Build history of the part. All positions in model axes, mm. A direction names the side the tool comes from. Give positions to 0.01 mm unless a question says otherwise; leave off trailing zeros. Write each loop counter-clockwise with the first axis right and the second up, starting at its lowest first coordinate (ties: lowest second). Pieces come first, ordered by that corner, then holes.
from build123d import *

# Parameters (mm, degrees)
SKETCH1_R                       = 1.5
BOSS_EXTRUDE1_DEPTH             = 2
SKETCH2_W                       = 4
SKETCH2_H                       = 25
BOSS_EXTRUDE2_DEPTH             = 15
FILLET1_R                       = 12.5
SKETCH3_R                       = 1.75
CUT_EXTRUDE3_DEPTH              = 53.391713426
CIRPATTERN1_COUNT               = 4
CIRPATTERN1_ANGLE               = 90
CIRPATTERN1_THE_OTHER_WAY_COUNT = 4
CIRPATTERN1_THE_OTHER_WAY_ANGLE = 90
MIRROR1_COPY_1_SKETCH_R         = 1.75
MIRROR1_COPY_1_DEPTH            = 53.391713426
MIRROR1_COPY_2_SKETCH_R         = 1.75
MIRROR1_COPY_2_DEPTH            = 53.391713426
MIRROR1_COPY_3_SKETCH_R         = 1.75
MIRROR1_COPY_3_DEPTH            = 53.391713426
MIRROR1_COPY_4_SKETCH_R         = 1.75
MIRROR1_COPY_4_DEPTH            = 53.391713426
MIRROR1_COPY_5_SKETCH_R         = 1.75
MIRROR1_COPY_5_DEPTH            = 53.391713426
MIRROR1_COPY_6_SKETCH_R         = 1.75
MIRROR1_COPY_6_DEPTH            = 53.391713426
FILLET1_OF_MIRROR1_R            = 12.5
SKETCH4_W                       = 30.151429758
SKETCH4_H                       = 10
BOSS_EXTRUDE3_DEPTH             = 7
FILLET2_R                       = 5


with BuildPart() as part:
    # Sketch1 → Boss-Extrude1 (new body)
    with BuildSketch(Plane(origin=(0, 0, 0), x_dir=(1, 0, 0), z_dir=(0, 1, 0))):
        with BuildLine():
            Line((-17.075714879, 5.179541619), (-17.075714879, 25.179541619))
            Line((-17.075714879, 25.179541619), (-26.075714879, 25.179541619))
            ThreePointArc((-26.075714879, 25.179541619), (-26.782821661, 24.8866484), (-27.075714879, 24.179541619))
            Line((-27.075714879, 24.179541619), (-27.075714879, -25.303833099))
            ThreePointArc((-27.075714879, -25.303833099), (-26.782821661, -26.010939881), (-26.075714879, -26.303833099))
            Line((-26.075714879, -26.303833099), (25.924285121, -26.303833099))
            ThreePointArc((25.924285121, -26.303833099), (26.631391902, -26.010939881), (26.924285121, -25.303833099))
            Line((26.924285121, -25.303833099), (26.924285121, 24.179541619))
            ThreePointArc((26.924285121, 24.179541619), (26.631391902, 24.8866484), (25.924285121, 25.179541619))
            Line((25.924285121, 25.179541619), (16.924285121, 25.179541619))
            Line((16.924285121, 25.179541619), (16.924285121, 5.179541619))
            ThreePointArc((16.924285121, 5.179541619), (15.459819027, 1.644007713), (11.924285121, 0.179541619))
            Line((11.924285121, 0.179541619), (-12.075714879, 0.179541619))
            ThreePointArc((-12.075714879, 0.179541619), (-15.611248785, 1.644007713), (-17.075714879, 5.179541619))
        make_face()
        with Locations(Location((-24.075714879, 22.179541619, 0), (0, 0, 270))):
            Circle(SKETCH1_R, mode=Mode.SUBTRACT)
        with Locations(Location((23.924285121, 22.179541619, 0), (0, 0, 270))):
            Circle(SKETCH1_R, mode=Mode.SUBTRACT)
        with Locations(Location((-24.075714879, -11.220458381, 0), (0, 0, 270))):
            Circle(SKETCH1_R, mode=Mode.SUBTRACT)
        with Locations(Location((-10.075714879, -22.220458381, 0), (0, 0, 270))):
            Circle(SKETCH1_R, mode=Mode.SUBTRACT)
        with Locations(Location((9.924285121, -22.220458381, 0), (0, 0, 270))):
            Circle(SKETCH1_R, mode=Mode.SUBTRACT)
        with Locations(Location((0, -20.835125629, 0), (0, 0, 270))):
            Circle(SKETCH1_R, mode=Mode.SUBTRACT)
        with Locations(Location((23.924285121, -11.220458381, 0), (0, 0, 270))):
            Circle(SKETCH1_R, mode=Mode.SUBTRACT)
    extrude(amount=BOSS_EXTRUDE1_DEPTH)

    # Sketch2 → Boss-Extrude2 (add)
    with BuildSketch(Plane(origin=(0, 2, 0), x_dir=(1, 0, 0), z_dir=(0, 1, 0))):
        with Locations((-17.075714879, -13.803833099)):
            Rectangle(SKETCH2_W, SKETCH2_H)
    boss_extrude2 = extrude(amount=BOSS_EXTRUDE2_DEPTH)

    # Fillet1
    fillet1_edges = [part.edges().sort_by_distance(p)[0] for p in [
        (-17.075714879, 17, 26.303833099),
        (-17.075714879, 17, 1.303833099),
    ]]
    fillet(fillet1_edges, radius=FILLET1_R - 0.0001)  # a hair under: the kernel refuses the full size

    # Sketch3 → Cut-Extrude3 (cut, through all)
    with BuildSketch(Plane(origin=(-15.075714879, 0, 0), x_dir=(0, 0, -1), z_dir=(1, 0, 0))):
        with Locations((-13.803833099, 14)):
            Circle(SKETCH3_R)
    cut_extrude3 = extrude(amount=-CUT_EXTRUDE3_DEPTH, mode=Mode.SUBTRACT)

    # CirPattern1: Cut-Extrude3 ×4 about axis
    cirpattern1_axis = Axis((0, 4.5, 13.803833099), (1, 0, 0))
    for i in range(1, CIRPATTERN1_COUNT):
        add(cut_extrude3.rotate(cirpattern1_axis, i * CIRPATTERN1_ANGLE / (CIRPATTERN1_COUNT - 1)), mode=Mode.SUBTRACT)

    # CirPattern1 the other way: Cut-Extrude3 ×4 about axis
    cirpattern1_the_other_way_axis = Axis((0, 4.5, 13.803833099), (-1, 0, 0))
    for i in range(1, CIRPATTERN1_THE_OTHER_WAY_COUNT):
        add(cut_extrude3.rotate(cirpattern1_the_other_way_axis, i * CIRPATTERN1_THE_OTHER_WAY_ANGLE / (CIRPATTERN1_THE_OTHER_WAY_COUNT - 1)), mode=Mode.SUBTRACT)

    # Mirror1: Boss-Extrude2, Cut-Extrude3 across plane
    add(boss_extrude2.mirror(Plane(origin=(0, 0, 0), x_dir=(0, 0, 1), z_dir=(1, 0, 0))))
    add(cut_extrude3.mirror(Plane(origin=(0, 0, 0), x_dir=(0, 0, 1), z_dir=(1, 0, 0))), mode=Mode.SUBTRACT)

    # Mirror1 copy 1 sketch → Mirror1 copy 1 (cut, through all)
    with BuildSketch(Plane(origin=(15.075714879, 7.504802233, -0.400637034), x_dir=(0, 0.5000000000000008, -0.8660254037844382), z_dir=(-1, 0, 0))):
        with Locations((-13.803833099, -14)):
            Circle(MIRROR1_COPY_1_SKETCH_R)
    extrude(amount=-MIRROR1_COPY_1_DEPTH, mode=Mode.SUBTRACT)

    # Mirror1 copy 2 sketch → Mirror1 copy 2 (cut, through all)
    with BuildSketch(Plane(origin=(15.075714879, 14.204470134, 3.004802233), x_dir=(0, 0.8660254037844396, -0.4999999999999984), z_dir=(-1, 0, 0))):
        with Locations((-13.803833099, -14)):
            Circle(MIRROR1_COPY_2_SKETCH_R)
    extrude(amount=-MIRROR1_COPY_2_DEPTH, mode=Mode.SUBTRACT)

    # Mirror1 copy 3 sketch → Mirror1 copy 3 (cut, through all)
    with BuildSketch(Plane(origin=(15.075714879, 18.303833099, 9.303833099), x_dir=(0, 1, 0), z_dir=(-1, 0, 0))):
        with Locations((-13.803833099, -14)):
            Circle(MIRROR1_COPY_3_SKETCH_R)
    extrude(amount=-MIRROR1_COPY_3_DEPTH, mode=Mode.SUBTRACT)

    # Mirror1 copy 4 sketch → Mirror1 copy 4 (cut, through all)
    with BuildSketch(Plane(origin=(15.075714879, -6.299030867, 4.099362966), x_dir=(0, -0.5000000000000008, -0.8660254037844382), z_dir=(-1, 0, 0))):
        with Locations((-13.803833099, -14)):
            Circle(MIRROR1_COPY_4_SKETCH_R)
    extrude(amount=-MIRROR1_COPY_4_DEPTH, mode=Mode.SUBTRACT)

    # Mirror1 copy 5 sketch → Mirror1 copy 5 (cut, through all)
    with BuildSketch(Plane(origin=(15.075714879, -9.704470134, 10.799030867), x_dir=(0, -0.8660254037844396, -0.4999999999999984), z_dir=(-1, 0, 0))):
        with Locations((-13.803833099, -14)):
            Circle(MIRROR1_COPY_5_SKETCH_R)
    extrude(amount=-MIRROR1_COPY_5_DEPTH, mode=Mode.SUBTRACT)

    # Mirror1 copy 6 sketch → Mirror1 copy 6 (cut, through all)
    with BuildSketch(Plane(origin=(15.075714879, -9.303833099, 18.303833099), x_dir=(0, -1, 0), z_dir=(-1, 0, 0))):
        with Locations((-13.803833099, -14)):
            Circle(MIRROR1_COPY_6_SKETCH_R)
    extrude(amount=-MIRROR1_COPY_6_DEPTH, mode=Mode.SUBTRACT)

    # Fillet1 of Mirror1
    fillet1_of_mirror1_edges = [part.edges().sort_by_distance(p)[0] for p in [
        (17.075714879, 17, 26.303833099),
        (17.075714879, 17, 1.303833099),
    ]]
    fillet(fillet1_of_mirror1_edges, radius=FILLET1_OF_MIRROR1_R - 0.0001)  # a hair under: the kernel refuses the full size

    # Sketch4 → Boss-Extrude3 (add)
    with BuildSketch(Plane(origin=(0, 2, 0), x_dir=(1, 0, 0), z_dir=(0, 1, 0))):
        with Locations((0, -12.553833099)):
            Rectangle(SKETCH4_W, SKETCH4_H)
    extrude(amount=BOSS_EXTRUDE3_DEPTH)

    # Fillet2
    fillet2_edges = [part.edges().sort_by_distance(p)[0] for p in [
        (0, 9, 17.553833099),
        (0, 9, 7.553833099),
    ]]
    fillet(fillet2_edges, radius=FILLET2_R - 0.0001)  # a hair under: the kernel refuses the full size


solid = part.part
1. Drop flat-ended pins along their axis: pin 1 (3 mm diameter, centred on y = 4.5, z = 4.3, fed in from -X); pin 2 (8 mm diameter, centred on x = -16, z = -8, fed in from +Y); pin 3 (7.5 mm diameter, centred on y = 9.5, z = 13, fed in from -X); pin 4 (2 mm diameter, centred on x = -2, y = 2.5, fed in from -Z). Give the stop position or say it passes through.
2. Mould opens along X. For faces 1 (the face through (19.076, 8, 14)), 2 (the face through (-27.076, 1, 0)), 3 (the face through (-17.05, 13.24, 22.74)), 4 (the face through (0, 3, 17.554)) say: pulls with the +X half, pulls with the -X half, needs draft (parallel to the pull), parting line crosses it, or undercut.
3. Drill centre lines: line 1 along Z through (x, y) = (-18.2, 4.5); line 2 along X through (y, z) = (16, 16); line 3 along Y through (x, z) = (18, 23.5). Where is each one in solid material? Low to high.
4. Saw through at B-B on z = -17. Give the cut face in (x, y), plus the area to 3 significant figures.
5. Saw through at D-D on z = -1. Give the cut face in (x, y), plus the area to 3 significant figures.
6. Saw through at C-C on x = 18. Count the separate pieces of the cut face and the enclosed holes in it, plus the area to 3 significant figures.
7. 3-axis set-ups, long thin cutter, end or side, ignore diameter. For faces 5 (the face through (0, 3, 7.554)), 6 (the face through (24.375, 0.986, -20.749)), 7 (the face through (-17.076, 1, -15)): which of +Z, -Z, +X, -X, +Y, -Y reach the whole face in a straight line?
Outcome:
1. pin 1: passes through
1. pin 2: stops at y = 2
1. pin 3: stops at x = -19.08
1. pin 4: stops at z = -0.18
2. face 1: pulls with the +X half
2. face 2: pulls with the -X half
2. face 3: needs draft
2. face 4: undercut
3. line 1: z = 1.3 to 2.55, 6.05 to 21.55, 25.05 to 26.3
3. line 2: x = -19.08 to -15.08, 15.08 to 19.08
3. line 3: y = 0 to 2.76, 6.24 to 8.3, 10.2 to 12.39
4. outline: (-27.08, 0) - (-17.08, 0) - (-17.08, 2) - (-27.08, 2) - close; (16.92, 0) - (26.92, 0) - (26.92, 2) - (16.92, 2) - close
4. area: 40.0 mm2
5. outline: (-27.08, 0) - (-14.82, 0) - (-14.82, 2) - (-27.08, 2) - close; (14.67, 0) - (26.92, 0) - (26.92, 2) - (14.67, 2) - close
5. area: 49.0 mm2
6. separate pieces: 1
6. enclosed holes: 7
6. area: 344 mm2
7. face 5: -Z, +Y
7. face 6: +Y, -Y
7. face 7: -Z, +Y, -Y
